from build123d import *

# Parameters (mm, degrees)
SKETCH1_W                                  = 70
SKETCH1_H                                  = 36
BOSS_EXTRUDE1_DEPTH                        = 8
SKETCH2_W                                  = 5.5
SKETCH2_H                                  = 8
CUT_EXTRUDE1_DEPTH                         = 41.162171256
CBORE_START                                = 33
CBORE_FOR_M3_CHEESE_HEAD_SCREW1_OUTLINE_R  = 3.25
CBORE_FOR_M3_CHEESE_HEAD_SCREW1_DEPTH      = 2
CBORE_START_2                              = 30.25
CBORE_FOR_M3_CHEESE_HEAD_SCREW1_2_OUTLIN_R = 1.7
CBORE_FOR_M3_CHEESE_HEAD_SCREW1_2_DEPTH    = 2.75
CUT_EXTRUDE2_DEPTH                         = 3


# Read off the part's stored shape, not the designer's step: CBORE for M3 Cheese Head Screw1
with BuildPart() as part:
    # Sketch1 → Boss-Extrude1 (new body)
    with BuildSketch(Plane(origin=(0, 0, 0), x_dir=(1, 0, 0), z_dir=(0, 1, 0))):
        Rectangle(SKETCH1_W, SKETCH1_H)
    extrude(amount=BOSS_EXTRUDE1_DEPTH)

    # Sketch2 → Cut-Extrude1 (cut, through all)
    with BuildSketch(Plane(origin=(0, 8, 0), x_dir=(1, 0, 0), z_dir=(0, 1, 0))):
        with Locations((-27.5, 14)):
            Rectangle(SKETCH2_W, SKETCH2_H)
        with Locations((27.5, 14)):
            Rectangle(SKETCH2_W, SKETCH2_H)
    extrude(amount=-CUT_EXTRUDE1_DEPTH, mode=Mode.SUBTRACT)

    # CBORE for M3 Cheese Head Screw1 outline → CBORE for M3 Cheese Head Screw1 (cut)
    with BuildSketch(Plane.YZ.offset(CBORE_START)):
        with Locations((4, -14)):
            Circle(CBORE_FOR_M3_CHEESE_HEAD_SCREW1_OUTLINE_R)
    cbore_for_m3_cheese_head_screw1 = extrude(amount=CBORE_FOR_M3_CHEESE_HEAD_SCREW1_DEPTH, mode=Mode.SUBTRACT)

    # CBORE for M3 Cheese Head Screw1 2 outlin → CBORE for M3 Cheese Head Screw1 2 (cut)
    with BuildSketch(Plane.YZ.offset(CBORE_START_2)):
        with Locations((4, -14)):
            Circle(CBORE_FOR_M3_CHEESE_HEAD_SCREW1_2_OUTLIN_R)
    cbore_for_m3_cheese_head_screw1_2 = extrude(amount=CBORE_FOR_M3_CHEESE_HEAD_SCREW1_2_DEPTH, mode=Mode.SUBTRACT)

    # Sketch9 → Cut-Extrude2 (cut)
    with BuildSketch(Plane(origin=(24.75, 0, 0), x_dir=(0, 0, -1), z_dir=(1, 0, 0))):
        Polygon((15.616580754, 6.8), (12.383419246, 6.8), (10.766838493, 4), (12.383419246, 1.2), (15.616580754, 1.2), (17.233161507, 4), align=None)
    cut_extrude2 = extrude(amount=-CUT_EXTRUDE2_DEPTH, mode=Mode.SUBTRACT)

    # Mirror1: CBORE for M3 Cheese Head Screw1, CBORE for M3 Cheese Head Screw1 2, Cut-Extrude2 across plane
    add(cbore_for_m3_cheese_head_screw1.mirror(Plane(origin=(0, 0, 0), x_dir=(0, 0, 1), z_dir=(1, 0, 0))), mode=Mode.SUBTRACT)
    add(cbore_for_m3_cheese_head_screw1_2.mirror(Plane(origin=(0, 0, 0), x_dir=(0, 0, 1), z_dir=(1, 0, 0))), mode=Mode.SUBTRACT)
    add(cut_extrude2.mirror(Plane(origin=(0, 0, 0), x_dir=(0, 0, 1), z_dir=(1, 0, 0))), mode=Mode.SUBTRACT)


solid = part.part
Here's how the part is built. I have some questions about the finished solid (model axes, mm). A direction names the side the tool comes from. Coordinates: 2 decimals unless noted, no trailing zeros. Order: outer loops, then holes, each group sorted by start corner. A loop starts at its lowest first (then second) coordinate and runs counter-clockwise, first axis right, second up.
Item 1: For P1, Ø3, axis at x = 28, y = 3, coming from the -Z side; P2, Ø1.7, axis at y = 3.5, z = -13, coming from the +X side; P3, Ø4, axis at y = 4, z = -14, coming from the -X side, each with a flat end and sliding along its axis, tell me the tip position at first contact or that it passes through.
Result sheet:
P1: stops at z = -10
P2: stops at x = 33
P3: stops at x = -33
Item 2: I need wall thicknesses on line 1 (Z direction, x = -30.95, y = 4); line 2 (Z direction, x = 34.1, y = 4); line 3 (X direction, y = 4.5, z = -14). Which ranges of each line are inside material? Lowest first, please.
Result sheet:
line 1: z = -18 to -15.7, -12.3 to 18
line 2: z = -18 to -17.25, -10.75 to 18
line 3: x = -21.75 to 21.75
Item 3: For faces 1 (the face through (33, 5.4, -15.4)), 2 (the face through (23.271, 5.38, -16.436)), 3 (the face through (30.25, 4, -12)), which set-ups out of +Z, -Z, +X, -X, +Y, -Y let a thin tool reach every point of the face, with its end or its side?
Result sheet:
face 1: +X
face 2: none
face 3: -Z, +Y, -Y
Item 4: If we section it at C-C on x = -27: List the corners of the cut face in (y, z) for me, plus the area to 3 significant figures.
Result sheet:
outline: (0, -10) - (8, -10) - (8, 18) - (0, 18) - close
area: 224 mm2
Item 5: If we section it at A-A on x = 24: List the corners of the cut face in (y, z) for me, plus the area to 3 significant figures.
Result sheet:
outline: (0, -18) - (8, -18) - (8, 18) - (0, 18) - close; hole (1.2, -15.62) - (4, -17.23) - (6.8, -15.62) - (6.8, -12.38) - (4, -10.77) - (1.2, -12.38) - close
area: 261 mm2
Item 6: If we mould it in two halves opening along Y, with no side actions, what happens to faces 4 (the face through (24.75, 5, -11)), 5 (the face through (-21.75, 4, -14)), 6 (the face through (0, 0, 0))? For each: +Y half, -Y half, draft (parallel to the pull), parting line (faces both ways), or undercut.
Result sheet:
face 4: draft
face 5: undercut
face 6: -Y half
Item 7: If we section it at B-B on z = -14: State how many separate pieces and enclosed holes the cut face has, plus the area to 3 significant figures.
Result sheet:
separate pieces: 5
enclosed holes: 0
area: 394 mm2
